Here's how the part is built. I have some questions about the finished solid (model axes, mm). Face numbers are marked on the shaded views. A direction names the side the tool comes from. Round coordinates to 2 decimals unless told otherwise and drop trailing zeros. Write each loop counter-clockwise with the first axis right and the second up, starting at its lowest first coordinate (ties: lowest second). Pieces come first, ordered by that corner, then holes. Notation, with made-up numbers: M 14,48 L 64,48 A19 ccw 64,58 Z; hole C 48.5,38.5 d2. An arc over 180 degrees is marked long. Use one line per item in the form item = value. Start each with the question number.
Q1. I want a section at A-A on y = 9.5. List the corners of the cut face in (x, z) for me, and give its area (3 significant figures).
Q2. I'm going to push flat-ended pins straight in: pin 1 Ø5 at (x, y) = (-22, 9) entering from +Z; pin 2 Ø1.2 at (y, z) = (5.5, 6) entering from +X; pin 3 Ø1.5 at (x, y) = (-20, 3) entering from -Z. Where does each tip first touch, or does it pass through?
Q3. I want a section at D-D on x = -23.5. List the corners of the cut face in (y, z) for me.
Q4. I need wall thicknesses on line 1 along X through (y, z) = (1.25, 1.75); line 2 along X through (y, z) = (7.5, 6.25); line 3 along Z through (x, y) = (-19.75, 1.25). Which ranges of each line are inside material? Lowest first, please. Write a range as from..to.
Q5. I want a section at B-B on z = 2. List the corners of the cut face in (x, y) for me.
Q6. For the marked faces 1, 2 and 3, which set-ups out of +Z, -Z, +X, -X, +Y, -Y let a thin tool reach every point of the face, with its end or its side?
Q7. I want a section at C-C on y = 5. List the corners of the cut face in (x, z) for me, and give its area (3 significant figures).
```python
from build123d import *

# Parameters (mm, degrees)
AUFSATZ_LINEAR_AUSTRAGEN1_DEPTH = 10
SKIZZE2_R                       = 1.25
AUFSATZ_LINEAR_AUSTRAGEN2_DEPTH = 2


with BuildPart() as part:
    # Skizze1 → Aufsatz-Linear austragen1 (new body)
    with BuildSketch(Plane(origin=(0, 0, 0), x_dir=(1, 0, 0), z_dir=(0, 1, 0))):
        Polygon((-16.813013293, -2.617875107), (-26.813013293, -5.297367031), (-26.813013293, -6.797367031), (-29.813013293, -6.797367031), (-29.813013293, 2.202632969), (-26.813013293, 2.202632969), (-26.813013293, 0.702632969), (-16.813013293, 0.702632969), align=None)
    extrude(amount=AUFSATZ_LINEAR_AUSTRAGEN1_DEPTH)

    # Skizze2 → Aufsatz-Linear austragen2 (add)
    with BuildSketch(Plane.ZY.offset(29.813013293)):
        with Locations((2.297367031, 5)):
            Circle(SKIZZE2_R)
    extrude(amount=AUFSATZ_LINEAR_AUSTRAGEN2_DEPTH)


solid = part.part
```
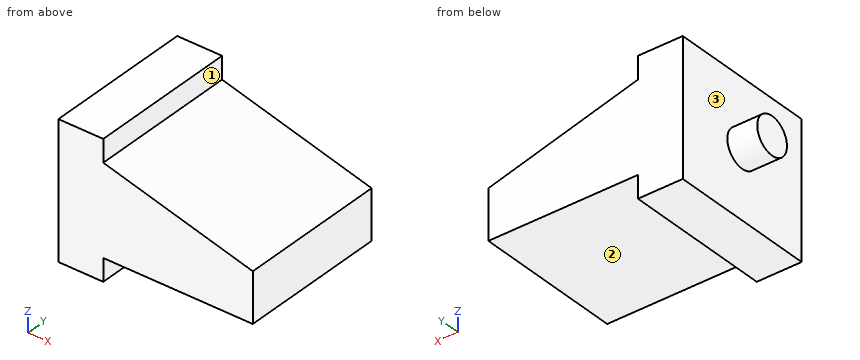
Reported:
q1.outline = M -29.81,-2.2 L -26.81,-2.2 L -26.81,-0.7 L -16.81,-0.7 L -16.81,2.62 L -26.81,5.3 L -26.81,6.8 L -29.81,6.8 Z
q1.area = 73.6 mm^2
q2.pin_1 = 4.68
q2.pin_2 = -26.81
q2.pin_3 = -0.7
q3.outline = M 0,-0.7 L 10,-0.7 L 10,4.41 L 0,4.41 Z
q4.line_1 = -29.81..-16.81
q4.line_2 = -29.81..-26.81
q4.line_3 = -0.7..3.4
q5.outline = M -31.81,3.79 L -29.81,3.79 L -29.81,0 L -16.81,0 L -16.81,10 L -29.81,10 L -29.81,6.21 L -31.81,6.21 Z
q6.face_1 = +Z, +X, +Y, -Y
q6.face_2 = -Z, +X, +Y, -Y
q6.face_3 = -X
q7.outline = M -31.81,1.05 L -29.81,1.05 L -29.81,-2.2 L -26.81,-2.2 L -26.81,-0.7 L -16.81,-0.7 L -16.81,2.62 L -26.81,5.3 L -26.81,6.8 L -29.81,6.8 L -29.81,3.55 L -31.81,3.55 Z
q7.area = 78.6 mm^2
